The drawing under review shows one solid part. Ordinate dimensions are in mm from its lowest x, y, z. Round coordinates to 2 decimals unless told otherwise and drop trailing zeros. Write each loop counter-clockwise with the first axis right and the second up, starting at its lowest first coordinate (ties: lowest second). Pieces come first, ordered by that corner, then holes. Notation, with made-up numbers: (25, 82) -> (62, 82) arc R31 ccw to (62, 121) -> close; hole circle Ø2 at (-16.5, -14.75). An arc over 180 degrees is marked (long way). Write item = value, one per line. Start each with the question number.
Item 1: Add section B-B, the plane x = 32. State the section outline as (y, z) points (3 decimals), then the cut area to 4 significant figures.
Item 2: Add section A-A, the plane z = 49. State the section outline as (x, y) points (3 decimals).
Item 3: For pin 1 Ø1 at (y, z) = (2, 1.5) entering from -X; pin 2 Ø1 at (y, z) = (1, 40) entering from +X, all flat-tipped, find the tip position at first contact; note any pin that passes through.
Item 4: Add section D-D, the plane z = 60.5. State the section outline as (x, y) points (3 decimals).
Item 5: Mouldability with a two-part tool opening along Y and no side actions: class the marked faces 1 and 2 as released by +Y, released by -Y, zero draft, split by the parting line, or undercut.
Item 6: Add section C-C, the plane x = 19.5. State the section outline as (y, z) points (3 decimals), then the cut area to 3 significant figures.
Item 7: To check wall thickness, follow L1, parallel to X at y = 0.15, z = 3 (3 decimals); L2, parallel to X at y = 0.2, z = 38.5 (3 decimals); L3, parallel to X at y = 0.2, z = 32 (3 decimals). State the ranges of each line that lie inside material, in increasing order.
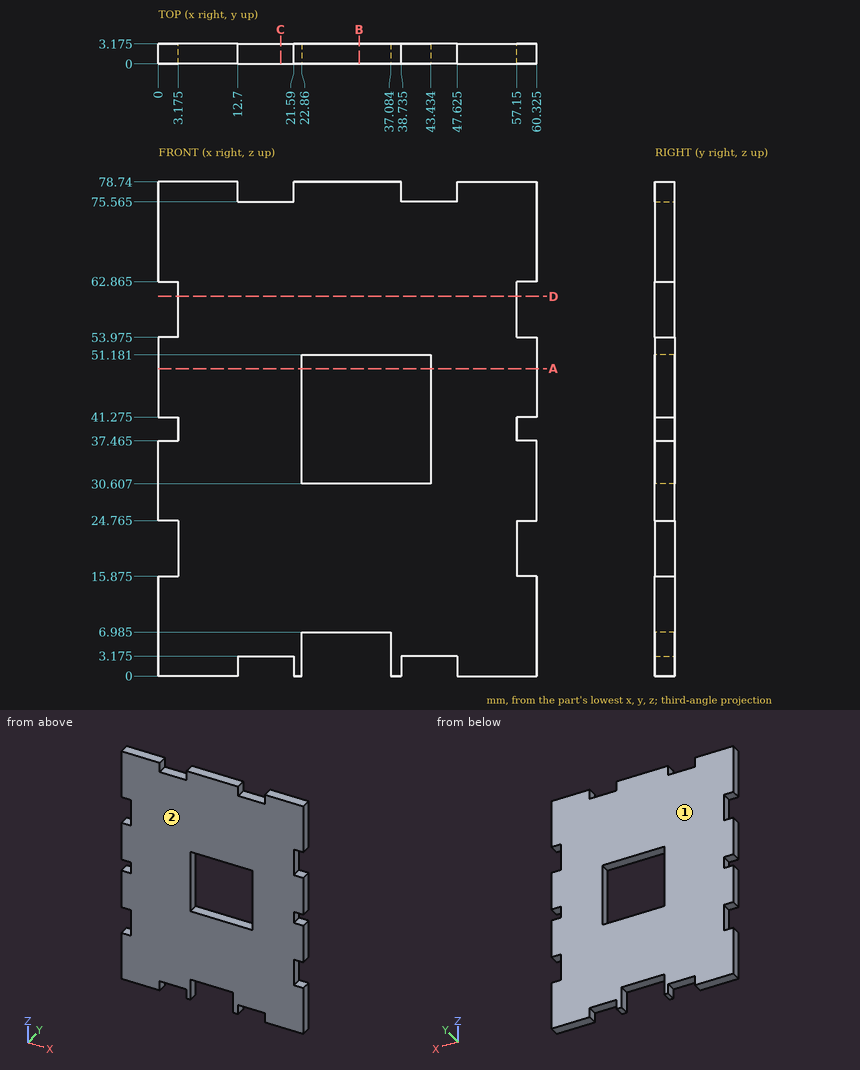
Result set:
q1.outline = (0, 6.985) -> (3.175, 6.985) -> (3.175, 30.607) -> (0, 30.607) -> close; (0, 51.181) -> (3.175, 51.181) -> (3.175, 78.74) -> (0, 78.74) -> close
q1.area = 162.5 mm²
q2.outline = (0, 0) -> (22.86, 0) -> (22.86, 3.175) -> (0, 3.175) -> close; (43.434, 0) -> (60.325, 0) -> (60.325, 3.175) -> (43.434, 3.175) -> close
q3.pin_1 = 0
q3.pin_2 = 57.15
q4.outline = (3.175, 0) -> (57.15, 0) -> (57.15, 3.175) -> (3.175, 3.175) -> close
q5.face_1 = released by +Y
q5.face_2 = released by -Y
q6.outline = (0, 3.175) -> (3.175, 3.175) -> (3.175, 75.565) -> (0, 75.565) -> close
q6.area = 230 mm²
q7.L1 = 0 to 12.7, 21.59 to 22.86, 37.084 to 38.735, 47.625 to 60.325
q7.L2 = 3.175 to 22.86, 43.434 to 57.15
q7.L3 = 0 to 22.86, 43.434 to 60.325
